Could you check a few things on this model? Use its own coordinates, in mm. A direction names the side the tool comes from. Coordinates: 2 decimals unless noted, no trailing zeros. Loops run counter-clockwise (first coordinate to the right, second up) from the corner with the lowest first, then second, coordinate; pieces in that order, holes last.
from build123d import *

# Parameters (mm, degrees)
CROQUIS2_W    = 1
CROQUIS2_H    = 1
CHAFL_N1_SIZE = 0.5


with BuildPart() as part:
    # Croquis1 → Revolución1 (revolve)
    with BuildSketch(Plane.XY, mode=Mode.PRIVATE) as revoluci_n1_sk:
        Polygon((0, 0), (-9.525, 0), (-9.525, 3), (-6, 3), (-6, 13), (-5, 13), (-5, 24), (0, 24), align=None)
    revolve(revoluci_n1_sk.sketch.rotate(Axis((0, 0, 0), (0, 1, 0)), 270), axis=Axis((0, 0, 0), (0, 1, 0)))

    # Croquis2 → Cortar-Revolución1 (revolve, cut)
    with BuildSketch(Plane.XY, mode=Mode.PRIVATE) as cortar_revoluci_n1_sk:
        with Locations((5, 21.5)):
            Rectangle(CROQUIS2_W, CROQUIS2_H)
    revolve(cortar_revoluci_n1_sk.sketch.rotate(Axis((0, 0, 0), (0, 1, 0)), 90), axis=Axis((0, 0, 0), (0, 1, 0)), mode=Mode.SUBTRACT)

    # Chaflán1
    chafl_n1_edges = [part.edges().sort_by_distance(p)[0] for p in [
        (0, 24, 5),
    ]]
    chamfer(chafl_n1_edges, length=CHAFL_N1_SIZE)


solid = part.part
(1) Imagine slicing it at A-A, the plane z = 0. Write out the boundary of the cut face in (x, y) (3 decimals).
Answers:
outline: (-9.525, 0) - (9.525, 0) - (9.525, 3) - (6, 3) - (6, 13) - (5, 13) - (5, 21) - (4.5, 21) - (4.5, 22) - (5, 22) - (5, 23.5) - (4.5, 24) - (-4.5, 24) - (-5, 23.5) - (-5, 22) - (-4.5, 22) - (-4.5, 21) - (-5, 21) - (-5, 13) - (-6, 13) - (-6, 3) - (-9.525, 3) - close
(2) Imagine slicing it at D-D, the plane y = 20.5. Write out the boundary of the cut face in (x, z), and give its area (3 significant figures).
Answers:
outline: circle Ø10 at (0, 0)
area: 78.5 mm2
(3) Imagine slicing it at B-B, the plane x = 0. Write out the boundary of the cut face in (y, z) (3 decimals), and give its area (3 significant figures).
Answers:
outline: (0, -9.525) - (3, -9.525) - (3, -6) - (13, -6) - (13, -5) - (21, -5) - (21, -4.5) - (22, -4.5) - (22, -5) - (23.5, -5) - (24, -4.5) - (24, 4.5) - (23.5, 5) - (22, 5) - (22, 4.5) - (21, 4.5) - (21, 5) - (13, 5) - (13, 6) - (3, 6) - (3, 9.525) - (0, 9.525) - close
area: 286 mm2
(4) Which directions (+Z, -Z, +X, -X, +Y, -Y) give clear straight access to the entire face, cutting with the end or side of a thin tool? Please do faces 1 (the face through (4.88, 22.76, 1.08)), 2 (the face through (0, 0, 0)).
Answers:
face 1: +Y
face 2: +Z, -Z, +X, -X, -Y
(5) For pin 1 (1 mm diameter, centred on y = 15.5, z = -2.5, fed in from -X); pin 2 (10 mm diameter, centred on x = 7, y = 9, fed in from -Z); pin 3 (6 mm diameter, centred on y = 19, z = -7, fed in from -X), each with a flat end and sliding along its axis, tell me the tip position at first contact or that it passes through.
Answers:
pin 1: stops at x = -4.58
pin 2: stops at z = -5.66
pin 3: stops at x = -3
(6) We'd pull the mould along Y, two halves only. Please class faces 3 (the face through (-3.04, 21.51, 3.32)), 4 (the face through (-4, 13, 4)), 5 (the face through (4.88, 17.06, 1.08)): +Y half, -Y half, draft (parallel to the pull), parting line (faces both ways), or undercut.
Answers:
face 3: undercut
face 4: +Y half
face 5: draft
(7) I need wall thicknesses on probe 1 along Y at (x, z) = (-5, -5.5); probe 2 along X at (y, z) = (2.75, 0) (3 decimals); probe 3 along Y at (x, z) = (-3.75, -4.5). Which ranges of each line are inside material? Lowest first, please.
Answers:
probe 1: y = 0 to 3
probe 2: x = -9.525 to 9.525
probe 3: y = 0 to 13
(8) Imagine slicing it at C-C, the plane y = 10.25. Write out the boundary of the cut face in (x, z).
Answers:
outline: circle Ø12 at (0, 0)
